Source: CAD feature listing. Evaluate the final solid. Frame: model axes, mm. A direction names the side the tool comes from. Give positions to 0.01 mm unless a question says otherwise; leave off trailing zeros. Write each loop counter-clockwise with the first axis right and the second up, starting at its lowest first coordinate (ties: lowest second). Pieces come first, ordered by that corner, then holes. Notation, with made-up numbers: M 65,89.25 L 89,89.25 A24 cw 89,119.25 Z; hole C -32,70.5 d2. An arc over 180 degrees is marked long. Return JSON: item names as keys, results as strings.
```python
from build123d import *

# Parameters (mm, degrees)
AUFSATZ_LINEAR_AUSTRAGEN1_DEPTH = 2.5
VERRUNDUNG1_R                   = 2
VERRUNDUNG2_R                   = 5
SKIZZE2_W                       = 60
SKIZZE2_H                       = 6
SCHNITT_LINEAR_AUSTRAGEN1_DEPTH = 1.7
SKIZZE3_W                       = 60
SKIZZE3_H                       = 2.5
AUFSATZ_LINEAR_AUSTRAGEN3_DEPTH = 2.3
SKIZZE5_R                       = 1
SCHNITT_LINEAR_AUSTRAGEN3_DEPTH = 2.5
SKIZZE6_R                       = 1
SCHNITT_LINEAR_AUSTRAGEN4_DEPTH = 2.5
SKIZZE7_W                       = 8
SKIZZE7_H                       = 8
SKIZZE7_R                       = 2
AUFSATZ_LINEAR_AUSTRAGEN4_DEPTH = 2.5
VERRUNDUNG3_R                   = 4
SKIZZE8_W                       = 1.041077985
SKIZZE8_H                       = 2.5
SCHNITT_LINEAR_AUSTRAGEN5_DEPTH = 0.6
SKIZZE10_W                      = 58.958922015
SKIZZE10_H                      = 0.6
SCHNITT_LINEAR_AUSTRAGEN6_DEPTH = 0.6
SCHNITT_LINEAR_AUSTRAGEN7_DEPTH = 1.6
SKIZZESTUTZENINNEN_R            = 2
AUFSATZ_LINEAR_AUSTRAGEN5_DEPTH = 2.5
VERRUNDUNG4_R                   = 1
VERRUNDUNG5_R                   = 2
VERRUNDUNG6_R                   = 2
SKIZZE12_R                      = 2
AUFSATZ_LINEAR_AUSTRAGEN6_DEPTH = 2.5
VERRUNDUNG7_R                   = 2
SKIZZE13_W                      = 1
SKIZZE13_H                      = 3.8
AUFSATZ_LINEAR_AUSTRAGEN7_DEPTH = 2.5
VERRUNDUNG9_R                   = 0.5


# Some blends are built 0.0001 mm under size
with BuildPart() as part:
    # d-body → Aufsatz-Linear austragen1 (new body)
    with BuildSketch(Plane.XY):
        with BuildLine():
            Line((25.141766665, 0), (-34.858233335, 0))
            Line((-34.858233335, 0), (-34.858233335, 15.8))
            ThreePointArc((-34.858233335, 15.8), (-31.050621491, 24.992388155), (-21.858233335, 28.8))
            ThreePointArc((-21.858233335, 28.8), (-17.008017348, 27.861318538), (-12.858233335, 25.18083152))
            Line((-12.858233335, 25.18083152), (0.141766665, 25.18083152))
            Line((0.141766665, 25.18083152), (0.141766665, 8))
            Line((0.141766665, 8), (25.141766665, 8))
            Line((25.141766665, 8), (25.141766665, 0))
        make_face()
    extrude(amount=AUFSATZ_LINEAR_AUSTRAGEN1_DEPTH)

    # Verrundung1
    verrundung1_edges = [part.edges().sort_by_distance(p)[0] for p in [
        (0.141766665, 25.18083152, 1.25),
    ]]
    fillet(verrundung1_edges, radius=VERRUNDUNG1_R)

    # Verrundung2
    verrundung2_edges = [part.edges().sort_by_distance(p)[0] for p in [
        (0.141766665, 8, 1.25),
    ]]
    fillet(verrundung2_edges, radius=VERRUNDUNG2_R)

    # Skizze2 → Schnitt-Linear austragen1 (cut)
    with BuildSketch(Plane.XY.offset(2.5)):
        with Locations((-4.858233335, 4)):
            Rectangle(SKIZZE2_W, SKIZZE2_H)
    extrude(amount=-SCHNITT_LINEAR_AUSTRAGEN1_DEPTH, mode=Mode.SUBTRACT)

    # Skizze3 → Aufsatz-Linear austragen3 (add)
    with BuildSketch(Plane.XY.offset(0.8)):
        with Locations((-4.858233335, 5.75)):
            Rectangle(SKIZZE3_W, SKIZZE3_H)
    extrude(amount=AUFSATZ_LINEAR_AUSTRAGEN3_DEPTH)

    # Skizze5 → Schnitt-Linear austragen3 (cut)
    with BuildSketch(Plane(origin=(0, 0, 0), x_dir=(-1, 0, 0), z_dir=(0, 0, -1))):
        with Locations((33.358233335, 9)):
            Circle(SKIZZE5_R)
    extrude(amount=-SCHNITT_LINEAR_AUSTRAGEN3_DEPTH, mode=Mode.SUBTRACT)

    # Skizze6 → Schnitt-Linear austragen4 (cut)
    with BuildSketch(Plane(origin=(0, 0, 0), x_dir=(-1, 0, 0), z_dir=(0, 0, -1))):
        with Locations((2.858233335, 9)):
            Circle(SKIZZE6_R)
    extrude(amount=-SCHNITT_LINEAR_AUSTRAGEN4_DEPTH, mode=Mode.SUBTRACT)

    # Skizze7 → Aufsatz-Linear austragen4 (add)
    with BuildSketch(Plane(origin=(0, 0, 0), x_dir=(-1, 0, 0), z_dir=(0, 0, -1))):
        with Locations((-29.141766665, 4)):
            Rectangle(SKIZZE7_W, SKIZZE7_H)
        with Locations((-29.141766665, 4)):
            Circle(SKIZZE7_R, mode=Mode.SUBTRACT)
    extrude(amount=-AUFSATZ_LINEAR_AUSTRAGEN4_DEPTH)

    # Verrundung3
    verrundung3_edges = [part.edges().sort_by_distance(p)[0] for p in [
        (33.141766665, 0, 1.25),
        (33.141766665, 8, 1.25),
    ]]
    fillet(verrundung3_edges, radius=VERRUNDUNG3_R - 0.0001)  # a hair under: the kernel refuses the full size

    # Skizze8 → Schnitt-Linear austragen5 (cut)
    with BuildSketch(Plane.XY.offset(3.1)):
        with Locations((24.621227673, 5.75)):
            Rectangle(SKIZZE8_W, SKIZZE8_H)
    extrude(amount=-SCHNITT_LINEAR_AUSTRAGEN5_DEPTH, mode=Mode.SUBTRACT)

    # Skizze10 → Schnitt-Linear austragen6 (cut)
    with BuildSketch(Plane.XY.offset(3.1)):
        with Locations((-5.378772328, 6.7)):
            Rectangle(SKIZZE10_W, SKIZZE10_H)
    extrude(amount=-SCHNITT_LINEAR_AUSTRAGEN6_DEPTH, mode=Mode.SUBTRACT)

    # Skizze11 → Schnitt-Linear austragen7 (cut)
    with BuildSketch(Plane.XY.offset(2.5)):
        with BuildLine():
            Line((-30.399734465, 9.324335962), (-5.252382746, 9.324335962))
            Line((-5.252382746, 9.324335962), (-5.252382746, 11.789002727))
            Line((-5.252382746, 11.789002727), (-1.923745725, 11.789002727))
            Line((-1.923745725, 11.789002727), (-1.923745725, 23.431190429))
            Line((-1.923745725, 23.431190429), (-13.163081736, 23.431190429))
            ThreePointArc((-13.163081736, 23.431190429), (-27.503142881, 25.898303071), (-32.913464689, 12.390808249))
            Line((-32.913464689, 12.390808249), (-32.913464689, 11.789002727))
            Line((-32.913464689, 11.789002727), (-30.399734465, 11.789002727))
            Line((-30.399734465, 11.789002727), (-30.399734465, 9.324335962))
        make_face()
    extrude(amount=-SCHNITT_LINEAR_AUSTRAGEN7_DEPTH, mode=Mode.SUBTRACT)

    # SkizzeStutzenInnen → Aufsatz-Linear austragen5 (add)
    # profile 1 of 2: a face of its own
    with BuildSketch(Plane.XY.offset(2.5)):
        with BuildLine():
            Line((-8.858233335, 25.18083152), (-8.858233335, 28.18083152))
            ThreePointArc((-8.858233335, 28.18083152), (-5.858233335, 31.18083152), (-2.858233335, 28.18083152))
            Line((-2.858233335, 28.18083152), (-2.858233335, 25.18083152))
            Line((-2.858233335, 25.18083152), (-8.858233335, 25.18083152))
        make_face()
        with Locations((-5.858233335, 28.18083152)):
            Circle(SKIZZESTUTZENINNEN_R, mode=Mode.SUBTRACT)
    # profile 2 of 2: a face of its own
    with BuildSketch(Plane.XY.offset(2.5)):
        with BuildLine():
            Line((-8.858233335, 0), (-8.858233335, -3))
            ThreePointArc((-8.858233335, -3), (-5.858233335, -6), (-2.858233335, -3))
            Line((-2.858233335, -3), (-2.858233335, 0))
            Line((-2.858233335, 0), (-8.858233335, 0))
        make_face()
        with Locations((-5.858233335, -3)):
            Circle(SKIZZESTUTZENINNEN_R, mode=Mode.SUBTRACT)
    extrude(amount=-AUFSATZ_LINEAR_AUSTRAGEN5_DEPTH)

    # Verrundung4
    # the kernel refuses this fillet: 1 mm, written as the material it adds along each edge
    with BuildSketch(Plane(origin=(-1.923745725, 23.431190429, 2.5), x_dir=(-1, 0, 0), z_dir=(0, 0, -1)), Plane(origin=(-1.923745725, 11.789002727, 2.5), x_dir=(0, 1, 0), z_dir=(0, 0, -1)), Plane(origin=(-5.252382746, 9.324335962, 2.5), x_dir=(0, 1, 0), z_dir=(0, 0, -1))) as verrundung4_piece_1:
        with BuildLine():
            CenterArc((VERRUNDUNG4_R, -VERRUNDUNG4_R), VERRUNDUNG4_R, 90, 90)
            Line((0, -VERRUNDUNG4_R), (0, 0))
            Line((0, 0), (VERRUNDUNG4_R, 0))
        make_face()
    extrude(amount=1.6)
    with BuildSketch(Plane(origin=(-32.913464689, 11.789002727, 2.5), x_dir=(1, 0, 0), z_dir=(0, 0, -1))) as verrundung4_piece_2:
        with BuildLine():
            CenterArc((0.917301018, -1), VERRUNDUNG4_R, 90, 66.534645017)
            Line((0, -0.601805522), (0, 0))
            Line((0, 0), (0.917301018, 0))
        make_face()
    extrude(amount=1.6)
    with BuildSketch(Plane(origin=(-30.399734465, 9.324335962, 2.5), x_dir=(0, 1, 0), z_dir=(0, 0, -1))) as verrundung4_piece_3:
        with BuildLine():
            CenterArc((VERRUNDUNG4_R, VERRUNDUNG4_R), VERRUNDUNG4_R, 180, 90)
            Line((0, VERRUNDUNG4_R), (0, 0))
            Line((0, 0), (VERRUNDUNG4_R, 0))
        make_face()
    extrude(amount=1.6)
    # the kernel refuses this fillet: 1 mm, written as the material it takes off along each edge
    with BuildSketch(Plane(origin=(-13.163081736, 23.431190429, 3.604131537), x_dir=(1, 0, 0), z_dir=(0, 0, -1))) as verrundung4_2_piece_1:
        with BuildLine():
            CenterArc((0.441652615, -1), VERRUNDUNG4_R, 90, 46.62999375)
            ThreePointArc((-0.28528164, -0.313292938), (-0.141206384, -0.157952653), (0, 0))
            Line((0, 0), (0.441652615, 0))
        make_face()
    extrude(amount=2.704131537, mode=Mode.SUBTRACT)
    with BuildSketch(Plane(origin=(-30.399734465, 11.789002727, 5), x_dir=(0, -1, 0), z_dir=(0, 0, -1))) as verrundung4_2_piece_2:
        with BuildLine():
            CenterArc((VERRUNDUNG4_R, VERRUNDUNG4_R), VERRUNDUNG4_R, 180, 90)
            Line((0, VERRUNDUNG4_R), (0, 0))
            Line((0, 0), (VERRUNDUNG4_R, 0))
        make_face()
    extrude(amount=4.1, mode=Mode.SUBTRACT)
    with BuildSketch(Plane(origin=(-5.252382746, 11.789002727, 5), x_dir=(0, -1, 0), z_dir=(0, 0, -1))) as verrundung4_2_piece_3:
        with BuildLine():
            CenterArc((VERRUNDUNG4_R, -VERRUNDUNG4_R), VERRUNDUNG4_R, 90, 90)
            Line((0, -VERRUNDUNG4_R), (0, 0))
            Line((0, 0), (VERRUNDUNG4_R, 0))
        make_face()
    extrude(amount=4.1, mode=Mode.SUBTRACT)

    # Verrundung5
    verrundung5_edges = [part.edges().sort_by_distance(p)[0] for p in [
        (-8.858233335, 0, 1.25),
        (-2.858233335, 0, 1.25),
        (-2.858233335, 25.18083152, 1.25),
        (-8.858233335, 25.18083152, 1.25),
    ]]
    fillet(verrundung5_edges, radius=VERRUNDUNG5_R)

    # Verrundung6
    verrundung6_edges = [part.edges().sort_by_distance(p)[0] for p in [
        (-12.858233335, 25.18083152, 1.25),
    ]]
    fillet(verrundung6_edges, radius=VERRUNDUNG6_R)

    # Skizze12 → Aufsatz-Linear austragen6 (add)
    with BuildSketch(Plane(origin=(0, 0, 0), x_dir=(-1, 0, 0), z_dir=(0, 0, -1))):
        with BuildLine():
            Line((28.858233335, 0), (34.858233335, 0))
            Line((34.858233335, 0), (34.858233335, -3))
            ThreePointArc((34.858233335, -3), (31.858233335, -6), (28.858233335, -3))
            Line((28.858233335, -3), (28.858233335, 0))
        make_face()
        with Locations((31.858233335, -3)):
            Circle(SKIZZE12_R, mode=Mode.SUBTRACT)
    extrude(amount=-AUFSATZ_LINEAR_AUSTRAGEN6_DEPTH)

    # Verrundung7
    verrundung7_edges = [part.edges().sort_by_distance(p)[0] for p in [
        (-28.858233335, 0, 1.25),
    ]]
    fillet(verrundung7_edges, radius=VERRUNDUNG7_R)

    # Skizze13 → Aufsatz-Linear austragen7 (add)
    with BuildSketch(Plane(origin=(0, 0, 0), x_dir=(-1, 0, 0), z_dir=(0, 0, -1))):
        with Locations((35.358233335, 8.9)):
            Rectangle(SKIZZE13_W, SKIZZE13_H)
    extrude(amount=-AUFSATZ_LINEAR_AUSTRAGEN7_DEPTH)

    # Verrundung9
    verrundung9_edges = [part.edges().sort_by_distance(p)[0] for p in [
        (-34.858233335, 10.8, 1.25),
        (-35.858233335, 7, 1.25),
        (-35.858233335, 10.8, 1.25),
    ]]
    fillet(verrundung9_edges, radius=VERRUNDUNG9_R - 0.0001)  # a hair under: the kernel refuses the full size


solid = part.part
```
1) Contact query for flat-ended pins moving along their axis: pin 1 Ø1.8 at (y, z) = (17, 2) entering from -X; pin 2 Ø0.5 at (y, z) = (-2.5, 1.5) entering from +X; pin 3 Ø0.8 at (x, z) = (18, 1) entering from -Y. Output: stop coordinate, or through.
Numbers:
{"pin 1": "stops at x = -34.85", "pin 2": "stops at x = -2.86", "pin 3": "stops at y = 0"}
2) Cut plane A-A, the plane x = -10. Return the cut outline in (y, z).
Numbers:
{"outline": "M -0.19,0 L 25.37,0 L 25.37,2.5 L 23.43,2.5 L 23.43,0.9 L 9.32,0.9 L 9.32,2.5 L 6.4,2.5 L 6.4,3.1 L 4.5,3.1 L 4.5,0.8 L 1,0.8 L 1,2.5 L -0.19,2.5 Z"}
3) Cut plane B-B, the plane z = 1.6. Give the number of separate pieces and of enclosed holes in the cut face, then the cut area to 3 significant figures.
Numbers:
{"separate pieces": "1", "enclosed holes": "7", "area": "546 mm²"}
4) Line query: line 1 (Y direction, x = -11, z = 0.85); line 2 (Z direction, x = 21, y = 4); line 3 (Y direction, x = -8, z = 2.2). Output: solid intervals per line, ascending. Write a range as [from, to].
Numbers:
{"line 1": "y = [0, 1], [4.5, 25.18]", "line 2": "z = [0, 0.8]", "line 3": "y = [-5.1, 1], [4.5, 9.32], [23.43, 30.28]"}
5) Set-up query: faces 1 (the face through (-34.858, 14, 1)), 2 (the face through (-9.43, 25.78, 1.23)), 3 (the face through (-28.288, -0.601, 1.268)), 4 (the face through (-8, 23.431, 2)), 5 (the face through (0.142, 18, 1)). Return all of +Z, -Z, +X, -X, +Y, -Y with unobstructed straight access to the full face (end or side cutting, diameter ignored); none if empty.
Numbers:
{"face 1": "+Z, -Z, -X, +Y", "face 2": "+Z, -Z, +Y", "face 3": "+Z, -Z, -Y", "face 4": "+Z", "face 5": "+Z, -Z, +X, +Y"}
